from build123d import *

# Parameters (mm, degrees)
SKETCH_1_W                     = 100
SKETCH_1_H                     = 7
EXTRUDE_1_DEPTH                = 4.8
HOLE_WIZARD_M1_6_1_D           = 2
HOLE_WIZARD_M1_6_1_CBORE_D     = 5
HOLE_WIZARD_M1_6_1_CBORE_DEPTH = 2


with BuildPart() as part:
    # 草图1 → 凸台-拉伸1 (new body)
    with BuildSketch(Plane(origin=(0, 4.8, 0), x_dir=(1, 0, 0), z_dir=(0, 1, 0))):
        Rectangle(SKETCH_1_W, SKETCH_1_H)
    extrude(amount=-EXTRUDE_1_DEPTH)

    # M1.6 凹头盖螺钉的柱形沉头孔1 (through all)
    with Locations(Plane(origin=(0, 4.8, 0), x_dir=(1, 0, 0), z_dir=(0, 1, 0))):
        with Locations((-30, 0), (-15, 0), (0, 0), (15, 0), (30, 0), (45, 0), (-45, 0)):
            CounterBoreHole(HOLE_WIZARD_M1_6_1_D / 2, HOLE_WIZARD_M1_6_1_CBORE_D / 2, HOLE_WIZARD_M1_6_1_CBORE_DEPTH)


solid = part.part
Read the model definition and answer for the solid it produces. Units are mm, in the model's axes. A direction names the side the tool comes from. Round coordinates to 2 decimals unless told otherwise and drop trailing zeros. Order: outer loops, then holes, each group sorted by start corner. A loop starts at its lowest first (then second) coordinate and runs counter-clockwise, first axis right, second up. Notation, with made-up numbers: (-36.75, 54) - (-31.75, 54) arc R8 cw to (-31.75, 65) - close; hole circle Ø9 at (35, 8.5). An arc over 180 degrees is marked (long way). Use one line per item in the form item = value. Start each with the question number.
(1) A flat-ended cylindrical pin translates along its axis: pin 1 Ø3 at (x, z) = (30, 0) entering from +Y. Find the tip coordinate at first contact, or state that the pin passes through.
(2) The part is cut by section A-A (y = 1.7). Give the vertices of the cut face in (x, z).
(3) Determine the mould class of faces 1 (the face through (-50, 2, 0)), 2 (the face through (-1, 2, 3.5)), 3 (the face through (1, 2.8, 1)) for opening direction Z: +Z half, -Z half, draft (parallel to the pull), parting line (faces both ways), or undercut.
(4) Find the intervals of material crossed by line 1 along Z through (x, y) = (45, 4.3); line 2 along Z through (x, y) = (45, 1.6); line 3 along Y through (x, z) = (2, -1), in increasing order. Write a range as from..to.
(5) The part is cut by section C-C (z = 0). Count the separate pieces of the cut face and the enclosed holes in it, then the cut area to 3 significant figures.
(6) For faces 4 (the face through (-29, 2.8, 1)), 5 (the face through (-29, 1, 0)), determine the directions among +Z, -Z, +X, -X, +Y, -Y from which every point of the face is accessible in a straight line to the end or side of a thin tool.
(7) The part is cut by section B-B (x = -45). Give the vertices of the cut face in (y, z), then the cut area to 3 significant figures.
Checked values:
q1.pin_1 = 2.8
q2.outline = (-50, -3.5) - (50, -3.5) - (50, 3.5) - (-50, 3.5) - close; hole circle Ø2 at (-45, 0); hole circle Ø2 at (-30, 0); hole circle Ø2 at (-15, 0); hole circle Ø2 at (0, 0); hole circle Ø2 at (15, 0); hole circle Ø2 at (30, 0); hole circle Ø2 at (45, 0)
q3.face_1 = draft
q3.face_2 = +Z half
q3.face_3 = undercut
q4.line_1 = -3.5..-2.5, 2.5..3.5
q4.line_2 = -3.5..-1, 1..3.5
q4.line_3 = 0..2.8
q5.separate_pieces = 8
q5.enclosed_holes = 0
q5.area = 371 mm^2
q6.face_4 = +Y
q6.face_5 = +Y, -Y
q7.outline = (0, -3.5) - (4.8, -3.5) - (4.8, -2.5) - (2.8, -2.5) - (2.8, -1) - (0, -1) - close; (0, 1) - (2.8, 1) - (2.8, 2.5) - (4.8, 2.5) - (4.8, 3.5) - (0, 3.5) - close
q7.area = 18.0 mm^2
